Part model, mm, in its own coordinate system. A direction names the side the tool comes from. Round coordinates to 2 decimals unless told otherwise and drop trailing zeros. Write each loop counter-clockwise with the first axis right and the second up, starting at its lowest first coordinate (ties: lowest second). Pieces come first, ordered by that corner, then holes. Notation, with made-up numbers: M 37.5,18.25 L 54.5,18.25 A23 cw 54.5,43.25 Z; hole C 62,17 d3. An arc over 180 degrees is marked long. One line per question, with ' | ' between items. Start each with the question number.
1) Saw through at C-C (x = -14.5). List the corners of the cut face in (y, z) (3 decimals).
2) Saw through at A-A (z = 2.55). Give the number of separate pieces and of enclosed holes in the cut face, plus the area to 3 significant figures.
3) Mould opens along Y. For faces 3 (the face through (-10.486, -9.137, 3.044)), 4 (the face through (-14, -4, 0)), 5 (the face through (-17.58, 4.032, 2.958)) say: pulls with the +Y half, pulls with the -Y half, needs draft (parallel to the pull), parting line crosses it, or undercut.
4) Drop flat-ended pins along their axis: pin 1 Ø1.8 at (y, z) = (-8.14, 3) entering from -X; pin 2 Ø1.3 at (y, z) = (-7.5, 3.5) entering from -X. Give the stop position or say it passes through.
5) Tool access for faces 1 (the face through (-9.5, -7, 2)), 2 (the face through (-11.5, -6.96, 3.03)): list every direction of +Z, -Z, +X, -X, +Y, -Y with a clear straight run to the whole face (end or side of a thin tool).
6) Wall check: probe 1 along Y at (x, z) = (-15, 2.9); probe 2 along Y at (x, z) = (-14.5, 5.45); probe 3 along X at (y, z) = (0.5, 4.6). Give the ranges that are in metal, low to high. Write a range as [from, to].
7) Saw through at B-B (y = -1). List the corners of the cut face in (x, z).
```python
from build123d import *

# Parameters (mm, degrees)
F0_R     = 2.475
F0_W     = 1.275
F0_H     = 4.75
F1_DEPTH = 6
F2_R     = 1
F3_DEPTH = 6.1501615181
F4_R     = 2.375
F4_R_2   = 1
F5_DEPTH = 2
F6_DEPTH = 2
F7_DEPTH = 25


with BuildPart() as f1:
    # F0 (on Top) → F1 (new body)
    with BuildSketch(Plane.XY):
        Polygon((-10.775, -9.0130328), (-12.4515975287, -9.0130328), (-10.775, -10.7171244104), align=None)
        with BuildLine():
            ThreePointArc((-18.4399316357, -2.9264975775), (-13.5543171095, -3.9293230017), (-10.775, 0.2119672))
            ThreePointArc((-10.775, 0.2119672), (-10.850506469, 1.0305523641), (-11.0744778417, 1.8215136285))
            ThreePointArc((-11.0744778417, 1.8215136285), (-17.6746133243, 3.9732004057), (-18.4399316357, -2.9264975775))
        make_face()
        with Locations((-15.25, 0.2119672)):
            Circle(F0_R, mode=Mode.SUBTRACT)
        with BuildLine():
            ThreePointArc((-11.0744778417, 1.8215136285), (-10.850506469, 1.0305523641), (-10.775, 0.2119672))
            Line((-10.775, 0.2119672), (-10.775, -4.2630328))
            Line((-10.775, -4.2630328), (-9.5, -4.2630328))
            Line((-9.5, -4.2630328), (-9.5, -2.2630328))
            Line((-9.5, -2.2630328), (-11.0744778417, 1.8215136285))
        make_face()
        with Locations((-10.1375, -6.6380328)):
            Rectangle(F0_W, F0_H)
        Polygon((-9.5, -9.0130328), (-10.775, -9.0130328), (-10.775, -10.7171244104), (-9.5, -12.0130328), align=None)
        with BuildLine():
            Line((-10.775, -4.2630328), (-10.775, 0.2119672))
            ThreePointArc((-10.775, 0.2119672), (-13.5543171095, -3.9293230017), (-18.4399316357, -2.9264975775))
            Line((-18.4399316357, -2.9264975775), (-12.4515975287, -9.0130328))
            Line((-12.4515975287, -9.0130328), (-10.775, -9.0130328))
            Line((-10.775, -9.0130328), (-10.775, -4.2630328))
        make_face()
    extrude(amount=F1_DEPTH)

    # F2 (on face) → F3 (cut, through all)
    with BuildSketch(Plane.YZ.offset(-9.5)):
        with BuildLine():
            ThreePointArc((-5.7630328, 3), (-8.1380328, 5.375), (-10.5130328, 3))
            ThreePointArc((-10.5130328, 3), (-8.1380328, 0.625), (-5.7630328, 3))
        make_face()
        with Locations((-8.1380328, 3)):
            Circle(F2_R, mode=Mode.SUBTRACT)
        with Locations((-8.1380328, 3)):
            Circle(F2_R)
    extrude(amount=-F3_DEPTH, mode=Mode.SUBTRACT)

    # F4 (on face) → F5 (join)
    with BuildSketch(Plane.YZ.offset(-9.5)):
        with Locations((-8.1380328, 3)):
            Circle(F4_R)
        with Locations((-8.1380328, 3)):
            Circle(F4_R_2, mode=Mode.SUBTRACT)
        with Locations((-8.1380328, 3)):
            Circle(F4_R_2)
    extrude(amount=-F5_DEPTH)

    # F4 (on face) → F6 (cut, through all)
    with BuildSketch(Plane.YZ.offset(-9.5)):
        with Locations((-8.1380328, 3)):
            Circle(F4_R_2)
    extrude(amount=-F6_DEPTH, mode=Mode.SUBTRACT)

    # F0 (on Top) → F7 (cut)
    with BuildSketch(Plane.XY):
        Polygon((-12.4515975287, -9.0130328), (-18.4399316357, -2.9264975775), (-21.0827792011, -5.5267050251), (-12.1428475655, -14.6132402476), (-9.5, -12.0130328), (-10.775, -10.7171244104), align=None)
    extrude(amount=F7_DEPTH, mode=Mode.SUBTRACT)


solid = f1.part
```
Answer key:
1) outline: M -6.931,0 L -2.147,0 L -2.147,6 L -6.931,6 L -6.931,5.045 A2.375 cw -6.931,0.955 Z; M 2.571,0 L 4.624,0 L 4.624,6 L 2.571,6 Z
2) separate pieces: 2 | enclosed holes: 1 | area: 70.5 mm2
3) face 3: undercut | face 4: needs draft | face 5: parting line crosses it
4) pin 1: passes through | pin 2: stops at x = -11.5
5) face 1: +Z, -Z, +X, +Y, -Y | face 2: -X
6) probe 1: y = [-5.77, -2.25], [2.67, 4.68] | probe 2: y = [-6.93, -2.15], [2.57, 4.62] | probe 3: x = [-19.72, -17.71], [-12.79, -10.57]
7) outline: M -19.56,0 L -17.41,0 L -17.41,6 L -19.56,6 Z; M -13.09,0 L -9.99,0 L -9.99,6 L -13.09,6 Z
